from build123d import *

# Parameters (mm, degrees)
EXTRUDE_2_DEPTH     = 1.5
SKETCH_2_R          = 1.5
CUT_EXTRUDE_1_DEPTH = 1.5
FILLET_3_R          = 0.15


with BuildPart() as part:
    # 草图1 → 凸台-拉伸2 (new body)
    with BuildSketch(Plane.XY):
        Polygon((0, 3.233161507), (-2.8, 1.616580754), (-2.8, -1.616580754), (0, -3.233161507), (2.8, -1.616580754), (2.8, 1.616580754), align=None)
    extrude(amount=-EXTRUDE_2_DEPTH)

    # 草图2 → 切除-拉伸1 (cut)
    with BuildSketch(Plane.XY):
        Circle(SKETCH_2_R)
    extrude(amount=-CUT_EXTRUDE_1_DEPTH, mode=Mode.SUBTRACT)

    # 圆角3
    fillet_3_edges = [part.edges().sort_by_distance(p)[0] for p in [
        (-1.5, 0, -1.5),
        (-1.5, 0, 0),
    ]]
    fillet(fillet_3_edges, radius=FILLET_3_R)

    # 草图3 → 切除-旋转1 (revolve, cut)
    with BuildSketch(Plane(origin=(0, 0, 0), x_dir=(0, 0, -1), z_dir=(1, 0, 0))):
        Polygon((0, 3.233161507), (0.41, 3.233161507), (0, 2.823161507), align=None)
        Polygon((1.5, 3.233161507), (1.09, 3.233161507), (1.5, 2.823161507), align=None)
    revolve(axis=Axis((0, 0, 0), (0, 0, -1)), mode=Mode.SUBTRACT)


solid = part.part
Can you work these out from the model? Positions are in its coordinate system, mm. Coordinates: 2 decimals unless noted, no trailing zeros. Write each loop counter-clockwise with the first axis right and the second up, starting at its lowest first coordinate (ties: lowest second). Pieces come first, ordered by that corner, then holes. Notation, with made-up numbers: (-39, 80.25) -> (-14, 80.25) arc R19 ccw to (-14, 84.25) -> close; hole circle Ø9 at (-6, 3.5). An arc over 180 degrees is marked (long way). Write item = value, one per line.
(1) Imagine slicing it at A-A (y = 0). Please give me the cut outline in (x, z), and give its area (3 significant figures).
Verdict:
outline = (-2.8, -1.5) -> (-1.65, -1.5) arc R0.15 ccw to (-1.5, -1.35) -> (-1.5, -0.15) arc R0.15 ccw to (-1.65, 0) -> (-2.8, 0) -> close; (1.5, -1.35) arc R0.15 ccw to (1.65, -1.5) -> (2.8, -1.5) -> (2.8, 0) -> (1.65, 0) arc R0.15 ccw to (1.5, -0.15) -> close
area = 3.88 mm^2
(2) Imagine slicing it at B-B (z = -0.8). Please give me the cut outline in (x, y).
Verdict:
outline = (-2.8, -1.62) -> (0, -3.23) -> (2.8, -1.62) -> (2.8, 1.62) -> (0, 3.23) -> (-2.8, 1.62) -> close; hole circle Ø3 at (0, 0)
(3) Thinking about a two-plate mould opening in X: for faces 1 (the face through (-1.42, -2.414, -0.74)), 2 (the face through (0, -2, 0)), 3 (the face through (-1.5, 0.07, -0.74)), 4 (the face through (2.8, 0, -1)), which applies, +X half, -X half, draft (parallel to the pull), parting line (faces both ways), or undercut?
Verdict:
face_1 = -X half
face_2 = draft
face_3 = undercut
face_4 = +X half
(4) If I drill on probe 1 along X at (y, z) = (-1.25, -0.6); probe 2 along X at (y, z) = (-0.5, -1.25); probe 3 along Y at (x, z) = (0.9, -0.1), over which ranges is the centre line in solid material (lowest first)?
Verdict:
probe_1 = -2.8 to -0.83, 0.83 to 2.8
probe_2 = -2.8 to -1.41, 1.41 to 2.8
probe_3 = -2.71 to -1.21, 1.21 to 2.71
(5) Imagine slicing it at C-C (y = 2.5). Please give me the cut outline in (x, z).
Verdict:
outline = (-1.27, -1.5) -> (1.27, -1.5) -> (1.27, 0) -> (-1.27, 0) -> close
